Here's how the part is built. I have some questions about the finished solid (model axes, mm). Face numbers are marked on the shaded views. A direction names the side the tool comes from. Coordinates: 2 decimals unless noted, no trailing zeros. Order: outer loops, then holes, each group sorted by start corner. A loop starts at its lowest first (then second) coordinate and runs counter-clockwise, first axis right, second up. Notation, with made-up numbers: (31, 62.5) - (60, 62.5) arc R19 cw to (60, 89.5) - close; hole circle Ø8 at (21, 67). An arc over 180 degrees is marked (long way). Answer in a Markdown table with one row per item. Add a question column.
Item 1: If I drill on line 1 along Y through (x, z) = (25.5, 0); line 2 along Z through (x, y) = (24, -4.5); line 3 along Y through (x, z) = (28, -0.5), over which ranges is the centre line in solid material (lowest first)? Write a range as from..to.
Item 2: I want a section at A-A (x = 19). Please give me the cut outline in (y, z).
Item 3: I want a section at B-B (x = 33). Please give me the cut outline in (y, z).
Item 4: On a 3-axis mill with a long thin cutter (end or side, diameter ignored), from which of +Z, -Z, +X, -X, +Y, -Y can I reach the whole of each face in a straight line? I mean the marked faces 4, 5, 6, 7 and 8. Say none if no direction works.
Item 5: Will these pins go through, and if not, where does the flat tip stop? pin 1 Ø0.6 at (x, y) = (-2, 0.5) entering from -Z; pin 2 Ø2 at (x, z) = (30, 15) entering from -Y; pin 3 Ø5 at (x, z) = (21, -1) entering from -Y.
Item 6: Thinking about a two-plate mould opening in Y: for the marked faces 1, 2 and 3, which applies, +Y half, -Y half, draft (parallel to the pull), parting line (faces both ways), or undercut?
```python
from build123d import *

# Parameters (mm, degrees)
SKETCH_8_W            = 12
SKETCH_8_H            = 10
EXTRUDE_1_DEPTH       = 24.3
SKETCH_10_R           = 1.5
EXTRUDE_2_DEPTH       = 5
SKETCH_11_R           = 2
EXTRUDE_3_DEPTH       = 0.8
SKETCH_12_R           = 2.5
EXTRUDE_4_DEPTH       = 1
SKETCH_13_R           = 22
EXTRUDE_1_2_DEPTH     = 9
SKETCH_15_R           = 14
CUT_EXTRUDE_3_DEPTH   = 4
SKETCH_16_R           = 22
SKETCH_16_R_2         = 14
EXTRUDE_7_DEPTH       = 9
SKETCH_17_W           = 2.3
SKETCH_17_H           = 12
CUT_EXTRUDE_3_2_DEPTH = 12
SKETCH_18_R           = 1
SKETCH_18_R_2         = 1.5
SKETCH_18_R_3         = 2.8
EXTRUDE_8_DEPTH       = 3
FILLET_1_R            = 3
FILLET_2_R            = 3
SKETCH_20_W           = 0.5
SKETCH_20_H           = 2
EXTRUDE_9_DEPTH       = 3
SKETCH_21_R           = 10.617088877
SKETCH_21_R_2         = 3.5
CUT_EXTRUDE_5_DEPTH   = 0.5


with BuildPart() as part:
    # Sketch 8 → Extrude 1 (new body)
    with BuildSketch(Plane(origin=(0, 0, 0), x_dir=(0, 0, -1), z_dir=(1, 0, 0))):
        Rectangle(SKETCH_8_W, SKETCH_8_H)
    extrude(amount=EXTRUDE_1_DEPTH)

    # Sketch 10 → Extrude 2 (add)
    with BuildSketch(Plane(origin=(24.3, 0, 0), x_dir=(0, 0, -1), z_dir=(1, 0, 0))):
        Circle(SKETCH_10_R)
    extrude(amount=EXTRUDE_2_DEPTH)

    # Sketch 11 → Extrude 3 (add)
    with BuildSketch(Plane(origin=(24.3, 0, 0), x_dir=(0, 0, -1), z_dir=(1, 0, 0))):
        with Locations((0.037058569, 0)):
            Circle(SKETCH_11_R)
    extrude(amount=EXTRUDE_3_DEPTH)

    # Sketch 12 → Extrude 4 (add)
    with BuildSketch(Plane.ZY):
        Circle(SKETCH_12_R)
    extrude(amount=EXTRUDE_4_DEPTH)

    # Sketch 13 → Extrude 1 2 (add)
    with BuildSketch(Plane(origin=(29.3, 0, 0), x_dir=(0, 0, -1), z_dir=(1, 0, 0))):
        Circle(SKETCH_13_R)
    extrude(amount=EXTRUDE_1_2_DEPTH)

    # Sketch 15 → Cut-Extrude 3 (cut)
    with BuildSketch(Plane(origin=(38.3, 0, 0), x_dir=(0, 0, -1), z_dir=(1, 0, 0))):
        Circle(SKETCH_15_R)
    extrude(amount=-CUT_EXTRUDE_3_DEPTH, mode=Mode.SUBTRACT)

    # Sketch 16 → Extrude 7 (add)
    with BuildSketch(Plane.ZY.offset(-29.3)):
        Circle(SKETCH_16_R)
        Circle(SKETCH_16_R_2, mode=Mode.SUBTRACT)
    extrude(amount=EXTRUDE_7_DEPTH)

    # Sketch 17 → Cut-Extrude 3 2 (cut)
    with BuildSketch(Plane(origin=(0, 5, 0), x_dir=(1, 0, 0), z_dir=(0, 1, 0))):
        with Locations((17.15, 0)):
            Rectangle(SKETCH_17_W, SKETCH_17_H)
    extrude(amount=-CUT_EXTRUDE_3_2_DEPTH, mode=Mode.SUBTRACT)


with BuildPart() as cut_extrude_3_2_piece_1:
    # of the separate pieces the step leaves, piece 1, a body of its own (cut_extrude_3_2_pieces)
    add(part.part.solids().sort_by_distance((29.3, 0, -22))[0])



with BuildPart() as cut_extrude_3_2_piece_2:
    # of the separate pieces the step leaves, piece 2, a body of its own (cut_extrude_3_2_pieces)
    add(part.part.solids().sort_by_distance((0, 5, 6))[0])


with BuildPart() as cut_extrude_3_2_piece_1_1:
    add(cut_extrude_3_2_piece_1.part)

    add(cut_extrude_3_2_piece_2.part)  # Extrude 8 merges Cut-Extrude 3 2 piece 2
    # Sketch 18 → Extrude 8 (add)
    with BuildSketch(Plane.ZY.offset(-18.3)):
        Circle(SKETCH_18_R)
        with Locations((3.6, 3)):
            Circle(SKETCH_18_R_2)
        with Locations((-3.6, -3)):
            Circle(SKETCH_18_R_2)
        with Locations(Location((-3.2, 2.2, 0), (0, 0, 180))):
            Circle(SKETCH_18_R_3)
    extrude(amount=EXTRUDE_8_DEPTH)

    # Fillet 1
    fillet_1_edges = [cut_extrude_3_2_piece_1_1.edges().sort_by_distance(p)[0] for p in [
        (38.3, 0, 22),
    ]]
    fillet(fillet_1_edges, radius=FILLET_1_R)

    # Fillet 2
    fillet_2_edges = [cut_extrude_3_2_piece_1_1.edges().sort_by_distance(p)[0] for p in [
        (20.3, 0, -22),
    ]]
    fillet(fillet_2_edges, radius=FILLET_2_R)

    # Sketch 20 → Extrude 9 (add)
    with BuildSketch(Plane.ZY):
        with Locations((3.75, 0)):
            Rectangle(SKETCH_20_W, SKETCH_20_H)
        with Locations((-3.75, 0)):
            Rectangle(SKETCH_20_W, SKETCH_20_H)
    extrude(amount=EXTRUDE_9_DEPTH)

    # Sketch 21 → Cut-Extrude 5 (cut)
    with BuildSketch(Plane(origin=(34.3, 0, 0), x_dir=(0, 0, -1), z_dir=(1, 0, 0))):
        Circle(SKETCH_21_R)
        Circle(SKETCH_21_R_2, mode=Mode.SUBTRACT)
    extrude(amount=-CUT_EXTRUDE_5_DEPTH, mode=Mode.SUBTRACT)


solid = cut_extrude_3_2_piece_1_1.part
```
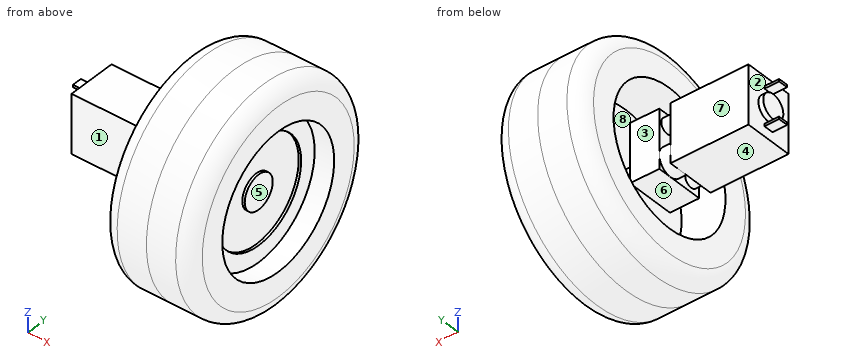
Values follow:
| question | item | result |
|---|---|---|
| 1 | line 1 | y = -22..-14, -1.5..1.5, 14..22 |
| 1 | line 2 | z = -21.53..-13.26, -6..6, 13.26..21.53 |
| 1 | line 3 | y = -21.99..-13.99, -1.41..1.41, 13.99..21.99 |
| 2 | outline | (-5, -6) - (5, -6) - (5, 6) - (-5, 6) - close |
| 3 | outline | circle Ø44 at (0, 0) |
| 4 | face 4 | -Z, -X, +Y, -Y |
| 4 | face 5 | +X |
| 4 | face 6 | -X |
| 4 | face 7 | +Z, -Z, -X, +Y |
| 4 | face 8 | none |
| 5 | pin 1 | stops at z = -4 |
| 5 | pin 2 | stops at y = -16.97 |
| 5 | pin 3 | stops at y = -22 |
| 6 | face 1 | -Y half |
| 6 | face 2 | draft |
| 6 | face 3 | undercut |
